Geometry: final body of the model. Coordinates: model frame, mm. A direction names the side the tool comes from. Round coordinates to 2 decimals unless told otherwise and drop trailing zeros. Loops run counter-clockwise (first coordinate to the right, second up) from the corner with the lowest first, then second, coordinate; pieces in that order, holes last. Notation, with made-up numbers: (33, 8.5) - (41, 8.5) arc R19 cw to (41, 23.5) - close; hole circle Ø10 at (45, 63.25). An arc over 180 degrees is marked (long way). Answer as a JSON object with one key per item and string values. Group by question number.
Item 1: Section C-C (x = 0). Return the cut outline in (y, z), plus the area to 3 significant figures.
Item 2: Line query: line 1 (X direction, y = 1.1, z = -30); line 2 (X direction, y = 4.25, z = 28); line 3 (Z direction, x = 0, y = 3.7). Output: solid intervals per line, ascending.
Item 3: Draft query along X for faces 3 (the face through (35, 5, -17)), 4 (the face through (27.56, 2.46, -40.25)). Return one class per face: released by +X, released by -X, zero draft, split by the parting line, or undercut.
Item 4: Reachability of faces 1 (the face through (-11.4, 7.5, 44.5)), 2 (the face through (-11.56, 2.46, 1.75)) from +Z, -Z, +X, -X, +Y, -Y: full face, straight path, thin tool, end or side. Return the list, or none.
Item 5: Section D-D (z = -30). Return the cut outline in (x, y).
Item 6: Section A-A (z = 28.35). Return the cut outline in (x, y), plus the area to 3 significant figures.
Item 7: Section B-B (y = 8.5). Return the cut outline in (x, z).
Item 8: First-contact query: pin 1 (3 mm diameter, centred on x = 22.5, y = 6, fed in from +Z); pin 2 (4 mm diameter, centred on y = 8.5, z = 56.5, fed in from +X); pin 3 (8 mm diameter, centred on x = -2, z = -8.5, fed in from -Y); pin 4 (9.5 mm diameter, centred on x = 0, z = -30, fed in from +Y). Flat tips, straight axial feed; report the tip coordinate or a pass-through.
```python
from build123d import *

# Parameters (mm, degrees)
BOSS_EXTRUDE1_DEPTH             = 10
CBORE_START                     = 5
CBORE_SLOT_FOR_M5_SHCS1_DEPTH   = 5
CBORE_SLOT_FOR_M5_SHCS1_2_DEPTH = 5
F_1_0MM_DOWEL_HOLE1_D           = 16.1
F_1_0MM_DOWEL_HOLE1_DEPTH       = 5.3
F_1_0MM_DOWEL_HOLE3_D           = 12
SKETCH14_R                      = 3.2
CUT_EXTRUDE1_DEPTH              = 77.249590163


# Read off the part's stored shape, not the designer's step: CBORE SLOT for M5 SHCS1
with BuildPart() as part:
    # Sketch1 → Boss-Extrude1 (new body)
    with BuildSketch(Plane(origin=(0, 0, 0), x_dir=(1, 0, 0), z_dir=(0, 1, 0))):
        Polygon((-25, 45), (35, 45), (35, -11), (2, -11), (2, -67), (-25, -67), align=None)
    extrude(amount=BOSS_EXTRUDE1_DEPTH)

    # CBORE SLOT for M5 SHCS1 outline → CBORE SLOT for M5 SHCS1 (cut)
    with BuildSketch(Plane(origin=(0, 0, 0), x_dir=(1, 0, 0), z_dir=(0, 1, 0)).offset(CBORE_START)):
        with BuildLine():
            Line((-6.5, -59.5), (-6.5, -49.5))
            ThreePointArc((-6.5, -49.5), (-11.5, -44.5), (-16.5, -49.5))
            Line((-16.5, -49.5), (-16.5, -59.5))
            ThreePointArc((-16.5, -59.5), (-11.5, -64.5), (-6.5, -59.5))
        make_face()
        with BuildLine():
            ThreePointArc((-6.5, 11), (-11.5, 16), (-16.5, 11))
            Line((-16.5, 11), (-16.5, 1))
            ThreePointArc((-16.5, 1), (-11.5, -4), (-6.5, 1))
            Line((-6.5, 1), (-6.5, 11))
        make_face()
        with BuildLine():
            Line((32.5, 27.5), (32.5, 37.5))
            ThreePointArc((32.5, 37.5), (27.5, 42.5), (22.5, 37.5))
            Line((22.5, 37.5), (22.5, 27.5))
            ThreePointArc((22.5, 27.5), (27.5, 22.5), (32.5, 27.5))
        make_face()
    extrude(amount=CBORE_SLOT_FOR_M5_SHCS1_DEPTH, mode=Mode.SUBTRACT)

    # CBORE SLOT for M5 SHCS1 2 outline → CBORE SLOT for M5 SHCS1 2 (cut)
    with BuildSketch(Plane(origin=(0, 0, 0), x_dir=(1, 0, 0), z_dir=(0, 1, 0))):
        with BuildLine():
            Line((-8.75, -59.5), (-8.75, -49.5))
            ThreePointArc((-8.75, -49.5), (-11.5, -46.75), (-14.25, -49.5))
            Line((-14.25, -49.5), (-14.25, -59.5))
            ThreePointArc((-14.25, -59.5), (-11.5, -62.25), (-8.75, -59.5))
        make_face()
        with BuildLine():
            ThreePointArc((-8.75, 11), (-11.5, 13.75), (-14.25, 11))
            Line((-14.25, 11), (-14.25, 1))
            ThreePointArc((-14.25, 1), (-11.5, -1.75), (-8.75, 1))
            Line((-8.75, 1), (-8.75, 11))
        make_face()
        with BuildLine():
            Line((30.25, 27.5), (30.25, 37.5))
            ThreePointArc((30.25, 37.5), (27.5, 40.25), (24.75, 37.5))
            Line((24.75, 37.5), (24.75, 27.5))
            ThreePointArc((24.75, 27.5), (27.5, 24.75), (30.25, 27.5))
        make_face()
    extrude(amount=CBORE_SLOT_FOR_M5_SHCS1_2_DEPTH, mode=Mode.SUBTRACT)

    # Ø1.0mm Dowel Hole1
    with Locations(Plane(origin=(0, 10, 0), x_dir=(1, 0, 0), z_dir=(0, 1, 0))):
        with Locations((0, 30)):
            Hole(F_1_0MM_DOWEL_HOLE1_D / 2, depth=F_1_0MM_DOWEL_HOLE1_DEPTH)

    # Ø1.0mm Dowel Hole3 (through all)
    with Locations(Plane(origin=(0, 4.7, 0), x_dir=(1, 0, 0), z_dir=(0, 1, 0))):
        with Locations((0, 30)):
            Hole(F_1_0MM_DOWEL_HOLE3_D / 2)

    # Sketch14 → Cut-Extrude1 (cut, through all)
    with BuildSketch(Plane(origin=(0, 10, 0), x_dir=(1, 0, 0), z_dir=(0, 1, 0))):
        with Locations((12, -28.35)):
            Circle(SKETCH14_R)
        with Locations(Location((-12, -28.35, 0), (0, 0, 270))):
            Circle(SKETCH14_R)
    extrude(amount=-CUT_EXTRUDE1_DEPTH, mode=Mode.SUBTRACT)


solid = part.part
```
Values:
{
 "1": {"outline": "(0, -45) - (10, -45) - (10, -38.05) - (4.7, -38.05) - (4.7, -36) - (0, -36) - close; (0, -24) - (4.7, -24) - (4.7, -21.95) - (10, -21.95) - (10, 67) - (0, 67) - close", "area": "978 mm^2"},
 "2": {"line 1": "x = -25 to -6, 6 to 24.75, 30.25 to 35", "line 2": "x = -25 to -15.18, -8.82 to 2", "line 3": "z = -45 to -36, -24 to 67"},
 "3": {"face 3": "released by +X", "face 4": "undercut"},
 "4": {"face 1": "+Y", "face 2": "+Y, -Y"},
 "5": {"outline": "(-25, 0) - (-6, 0) - (-6, 4.7) - (-8.05, 4.7) - (-8.05, 10) - (-25, 10) - close; (6, 0) - (24.75, 0) - (24.75, 5) - (22.5, 5) - (22.5, 10) - (8.05, 10) - (8.05, 4.7) - (6, 4.7) - close; (30.25, 0) - (35, 0) - (35, 10) - (32.5, 10) - (32.5, 5) - (30.25, 5) - close"},
 "6": {"outline": "(-25, 0) - (-15.2, 0) - (-15.2, 10) - (-25, 10) - close; (-8.8, 0) - (2, 0) - (2, 10) - (-8.8, 10) - close", "area": "206 mm^2"},
 "7": {"outline": "(-25, -45) - (35, -45) - (35, 11) - (2, 11) - (2, 67) - (-25, 67) - close; hole (-16.5, -11) arc R5 ccw to (-6.5, -11) - (-6.5, -1) arc R5 ccw to (-16.5, -1) - close; hole (-16.5, 49.5) arc R5 ccw to (-6.5, 49.5) - (-6.5, 59.5) arc R5 ccw to (-16.5, 59.5) - close; hole circle Ø6.4 at (-12, 28.35); hole circle Ø16.1 at (0, -30); hole (22.5, -37.5) arc R5 ccw to (32.5, -37.5) - (32.5, -27.5) arc R5 ccw to (22.5, -27.5) - close"},
 "8": {"pin 1": "stops at z = 11", "pin 2": "stops at x = 2", "pin 3": "stops at y = 0", "pin 4": "passes through"}
}
